```python
from build123d import *

# Parameters (mm, degrees)
F0_W     = 47.5
F0_H     = 35
F1_DEPTH = 17.5
F2_W     = 37.100266
F2_H     = 10
F3_DEPTH = 35.001
F5_DEPTH = 47.501
F6_W     = 22.5
F6_H     = 4
F7_DEPTH = 7.501


with BuildPart() as f1:
    # F0 (on Top) → F1 (new body)
    with BuildSketch(Plane.XY):
        with Locations((-6.113795, 9.902082)):
            Rectangle(F0_W, F0_H)
    extrude(amount=F1_DEPTH)

    # F2 (on face) → F3 (cut, through all)
    with BuildSketch(Plane.XZ.offset(7.597918)):
        with Locations((-0.913928, 12.5)):
            Rectangle(F2_W, F2_H)
    extrude(amount=-F3_DEPTH, mode=Mode.SUBTRACT)

    # F4 (on face) → F5 (cut, through all)
    with BuildSketch(Plane(origin=(-29.863795, 0, 0), x_dir=(0, -1, 0), z_dir=(-1, 0, 0))):
        Polygon((-19.902082, 17.5), (-22.402082, 12.5), (2.597918, 12.5), (0.097918, 17.5), align=None)
    extrude(amount=-F5_DEPTH, mode=Mode.SUBTRACT)

    # F6 (on face) → F7 (cut, through all)
    with BuildSketch(Plane.XY.offset(7.5)):
        Polygon((5.136205, -7.597918), (17.636205, -7.597918), (17.636205, 4.74937), align=None)
        Polygon((17.636205, 27.402082), (5.136205, 27.402082), (17.636205, 13.74937), align=None)
        with Locations((6.386205, 9.24937)):
            Rectangle(F6_W, F6_H)
    extrude(amount=-F7_DEPTH, mode=Mode.SUBTRACT)


solid = f1.part
```
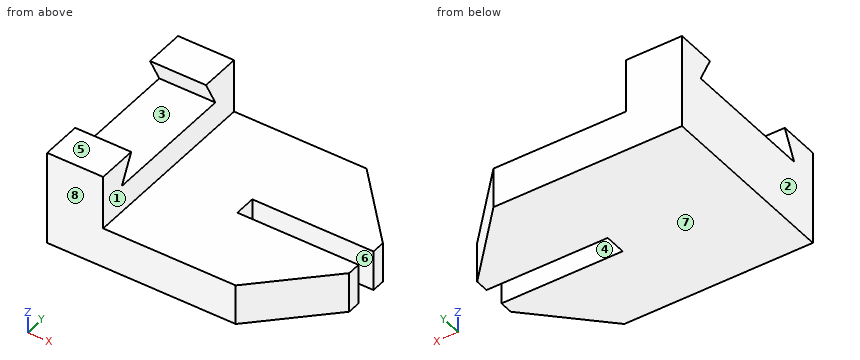
Here's how the part is built. I have some questions about the finished solid (model axes, mm). Face numbers are marked on the shaded views. A direction names the side the tool comes from. Coordinates: 2 decimals unless noted, no trailing zeros. Write each loop counter-clockwise with the first axis right and the second up, starting at its lowest first coordinate (ties: lowest second). Pieces come first, ordered by that corner, then holes. Notation, with made-up numbers: (33.25, 16) - (62.25, 16) arc R34 ccw to (62.25, 47) - close; hole circle Ø4 at (64.5, 64). An arc over 180 degrees is marked (long way). One line per item, written item: value.
1) Suppose I cut it at B-B on x = 7. Write out the boundary of the cut face in (y, z), and give its area (3 significant figures).
Model answer:
outline: (-5.76, 0) - (7.25, 0) - (7.25, 7.5) - (-5.76, 7.5) - close; (11.25, 0) - (25.37, 0) - (25.37, 7.5) - (11.25, 7.5) - close
area: 203 mm²
2) Suppose I cut it at A-A on z = 13.5. Write out the boundary of the cut face in (x, y), and give its area (3 significant figures).
Model answer:
outline: (-29.86, -7.6) - (-19.46, -7.6) - (-19.46, -2.1) - (-29.86, -2.1) - close; (-29.86, 21.9) - (-19.46, 21.9) - (-19.46, 27.4) - (-29.86, 27.4) - close
area: 114 mm²
3) Suppose I cut it at D-D on z = 4.75. Write out the boundary of the cut face in (x, y), and give its area (3 significant figures).
Model answer:
outline: (-29.86, -7.6) - (5.14, -7.6) - (17.64, 4.75) - (17.64, 7.25) - (-4.86, 7.25) - (-4.86, 11.25) - (17.64, 11.25) - (17.64, 13.75) - (5.14, 27.4) - (-29.86, 27.4) - close
area: 1,410 mm²
4) We'd pull the mould along Y, two halves only. Please class the marked faces 6, 7 and 8: pulls with the +Y half, pulls with the -Y half, needs draft (parallel to the pull), parting line crosses it, or undercut.
Model answer:
face 6: undercut
face 7: needs draft
face 8: pulls with the -Y half
5) I'm going to push flat-ended pins straight in: P1, Ø5, axis at x = -14, y = 12.5, coming from the +Z side; P2, Ø3, axis at x = -23.5, y = 10.5, coming from the +Z side; P3, Ø2, axis at x = 9, z = 3, coming from the -Y side. Where does each tip first touch, or does it pass through?
Model answer:
P1: stops at z = 7.5
P2: stops at z = 12.5
P3: stops at y = -4.77
6) I need wall thicknesses on line 1 along Y through (x, z) = (0.5, 5); line 2 along X through (y, z) = (-3, 13.25); line 3 along Z through (x, y) = (-17, 1.5). Which ranges of each line are inside material? Lowest first, please.
Model answer:
line 1: y = -7.6 to 7.25, 11.25 to 27.4
line 2: x = -29.86 to -19.46
line 3: z = 0 to 7.5
7) On a 3-axis mill with a long thin cutter (end or side, diameter ignored), from which of +Z, -Z, +X, -X, +Y, -Y can I reach the whole of each face in a straight line? I mean the marked faces 1, 2, 3, 4 and 5. Say none if no direction works.
Model answer:
face 1: +Z, +X, +Y, -Y
face 2: +Z, -Z, -X, +Y, -Y
face 3: +X, -X
face 4: +Z, -Z, +X
face 5: +Z, +X, -X, +Y, -Y
8) Suppose I cut it at C-C on y = 8. Write out the boundary of the cut face in (x, z).
Model answer:
outline: (-29.86, 0) - (-4.86, 0) - (-4.86, 7.5) - (-19.46, 7.5) - (-19.46, 12.5) - (-29.86, 12.5) - close
